Geometry check sheet. Reference: the model listing, model coordinates, mm. A direction names the side the tool comes from. Give positions to 0.01 mm unless a question says otherwise; leave off trailing zeros. Loops run counter-clockwise (first coordinate to the right, second up) from the corner with the lowest first, then second, coordinate; pieces in that order, holes last. Notation, with made-up numbers: (33.5, 61.25) - (80.5, 61.25) arc R25 cw to (80.5, 74.25) - close; hole circle Ø8 at (-25, 49). An arc over 180 degrees is marked (long way). Use a Markdown table: item, result. Add a question column.
1. Cross-section at D-D on y = 9.25. Enter the section's corners in (x, z), and give its area (3 significant figures).
2. Draft check along Z on faces 1 (the flat face through (4, 0, 9)), 2 (the flat face through (2, 10, 2.964)), 3 (the flat face through (4, 10, 27.464)). Enter one of: pulls with the +Z half, pulls with the -Z half, needs draft (parallel to the pull), parting line crosses it, or undercut.
3. Cross-section at B-B on y = 15. Enter the section's corners in (x, z), and give its area (3 significant figures).
4. Cross-section at C-C on z = 16.5. Enter the section's corners in (x, y).
5. Material ranges on L1, parallel to Z at x = 1.75, y = 18.5; L2, parallel to Z at x = 1.75, y = 8.25; L3, parallel to Y at x = 2.5, z = -8, recorded low to high.
6. Cross-section at A-A on x = 3.5. Enter the section's corners in (y, z).
7. Set-up check for faces 4 (the flat face through (0.5, 12, 15)), 5 (the flat face through (2, 10, -5.036)), 6 (the cylindrical face through (3.704, 7.782, 18.618)): record each of +Z, -Z, +X, -X, +Y, -Y from which the full face is reachable in a straight line by a thin tool's end or side.
8. Depth check by flat-ended pin: P1, Ø12, axis at y = 10.5, z = 23, coming from the -X side; P2, Ø2.5, axis at y = 7, z = 0, coming from the -X side; P3, Ø1.5, axis at y = 10, z = 16.5, coming from the +X side. Enter the tip coordinate at first touch or a pass-through.
from build123d import *

# Parameters (mm, degrees)
BOSS_EXTRUDE1_DEPTH = 20
CUT_EXTRUDE1_REACH  = 25.446
SKETCH2_R           = 1.3
SKETCH4_W           = 6.5
SKETCH4_H           = 21.5
BOSS_EXTRUDE2_DEPTH = 20
CUT_EXTRUDE2_REACH  = 36.591
SKETCH6_R           = 1.3
CUT_EXTRUDE3_REACH  = 36.591
SKETCH7_R           = 2.5


with BuildPart() as part:
    # Sketch1 → Boss-Extrude1 (new body)
    with BuildSketch(Plane(origin=(0, 0, 0), x_dir=(-1, 0, 0), z_dir=(0, 1, 0))):
        Polygon((0, -5.035714286), (0, -10.035714286), (-7, -10.035714286), (-7, 5.964285714), (-0.5, 5.964285714), (-0.5, 2.964285714), (-4, 2.964285714), (-4, -5.035714286), align=None)
    extrude(amount=BOSS_EXTRUDE1_DEPTH)

    # Sketch2 → Cut-Extrude1 (cut, up to next)
    with BuildSketch(Plane(origin=(0, 0, 0), x_dir=(0, -1, 0), z_dir=(-1, 0, 0)), mode=Mode.PRIVATE) as cut_extrude1_sk1:
        with Locations(Location((-15, -7.535714286, 0), (0, 0, 90))):
            Circle(SKETCH2_R)
    cut_extrude1_tool1 = extrude(cut_extrude1_sk1.sketch, amount=-CUT_EXTRUDE1_REACH, mode=Mode.PRIVATE) & part.part
    # Sketch2 → Cut-Extrude1 (cut, up to next)
    with BuildSketch(Plane(origin=(0, 0, 0), x_dir=(0, -1, 0), z_dir=(-1, 0, 0)), mode=Mode.PRIVATE) as cut_extrude1_sk2:
        with Locations(Location((-5, -7.535714286, 0), (0, 0, 90))):
            Circle(SKETCH2_R)
    cut_extrude1_tool2 = extrude(cut_extrude1_sk2.sketch, amount=-CUT_EXTRUDE1_REACH, mode=Mode.PRIVATE) & part.part
    add(cut_extrude1_tool1.solids().sort_by_distance((0, 15, -7.535714))[0], mode=Mode.SUBTRACT)
    add(cut_extrude1_tool2.solids().sort_by_distance((0, 5, -7.535714))[0], mode=Mode.SUBTRACT)

    # Sketch4 → Boss-Extrude2 (add)
    with BuildSketch(Plane(origin=(0, 20, 0), x_dir=(-1, 0, 0), z_dir=(0, 1, 0))):
        with Locations((-3.75, 16.714285714)):
            Rectangle(SKETCH4_W, SKETCH4_H)
    extrude(amount=-BOSS_EXTRUDE2_DEPTH)

    # Sketch6 → Cut-Extrude2 (cut, up to next)
    with BuildSketch(Plane(origin=(0.5, 0, 0), x_dir=(0, -1, 0), z_dir=(-1, 0, 0)), mode=Mode.PRIVATE) as cut_extrude2_sk1:
        with Locations(Location((-15, 5.464285714, 0), (0, 0, 90))):
            Circle(SKETCH6_R)
    cut_extrude2_tool1 = extrude(cut_extrude2_sk1.sketch, amount=-CUT_EXTRUDE2_REACH, mode=Mode.PRIVATE) & part.part
    # Sketch6 → Cut-Extrude2 (cut, up to next)
    with BuildSketch(Plane(origin=(0.5, 0, 0), x_dir=(0, -1, 0), z_dir=(-1, 0, 0)), mode=Mode.PRIVATE) as cut_extrude2_sk2:
        with Locations(Location((-5, 5.464285714, 0), (0, 0, 90))):
            Circle(SKETCH6_R)
    cut_extrude2_tool2 = extrude(cut_extrude2_sk2.sketch, amount=-CUT_EXTRUDE2_REACH, mode=Mode.PRIVATE) & part.part
    add(cut_extrude2_tool1.solids().sort_by_distance((0.5, 15, 5.464286))[0], mode=Mode.SUBTRACT)
    add(cut_extrude2_tool2.solids().sort_by_distance((0.5, 5, 5.464286))[0], mode=Mode.SUBTRACT)

    # Sketch7 → Cut-Extrude3 (cut, up to next)
    with BuildSketch(Plane(origin=(0.5, 0, 0), x_dir=(0, -1, 0), z_dir=(-1, 0, 0)), mode=Mode.PRIVATE) as cut_extrude3_sk1:
        with Locations(Location((-10, 17.464285714, 0), (0, 0, 90))):
            Circle(SKETCH7_R)
    cut_extrude3_tool1 = extrude(cut_extrude3_sk1.sketch, amount=-CUT_EXTRUDE3_REACH, mode=Mode.PRIVATE) & part.part
    add(cut_extrude3_tool1.solids().sort_by_distance((0.5, 10, 17.464286))[0], mode=Mode.SUBTRACT)


solid = part.part
Values found:
| question | item | result |
|---|---|---|
| 1 | outline | (0, -10.04) - (7, -10.04) - (7, 15.08) - (0.5, 15.08) - (0.5, 2.96) - (4, 2.96) - (4, -5.04) - (0, -5.04) - close; (0.5, 19.85) - (7, 19.85) - (7, 27.46) - (0.5, 27.46) - close |
| 1 | area | 187 mm2 |
| 2 | face 1 | needs draft |
| 2 | face 2 | undercut |
| 2 | face 3 | pulls with the +Z half |
| 3 | outline | (0, -10.04) - (7, -10.04) - (7, -8.84) - (0, -8.84) - close; (0, -6.24) - (7, -6.24) - (7, 4.16) - (0.5, 4.16) - (0.5, 2.96) - (4, 2.96) - (4, -5.04) - (0, -5.04) - close; (0.5, 6.76) - (7, 6.76) - (7, 27.46) - (0.5, 27.46) - close |
| 3 | area | 183 mm2 |
| 4 | outline | (0.5, 0) - (7, 0) - (7, 7.69) - (0.5, 7.69) - close; (0.5, 12.31) - (7, 12.31) - (7, 20) - (0.5, 20) - close |
| 5 | L1 | z = -10.04 to -5.04, 2.96 to 27.46 |
| 5 | L2 | z = -10.04 to -5.04, 2.96 to 15.68, 19.25 to 27.46 |
| 5 | L3 | y = 0 to 3.79, 6.21 to 13.79, 16.21 to 20 |
| 6 | outline | (0, -10.04) - (20, -10.04) - (20, -5.04) - (0, -5.04) - close; (0, 2.96) - (20, 2.96) - (20, 27.46) - (0, 27.46) - close; hole circle Ø2.6 at (5, -7.54); hole circle Ø2.6 at (5, 5.46); hole circle Ø5 at (10, 17.46); hole circle Ø2.6 at (15, -7.54); hole circle Ø2.6 at (15, 5.46) |
| 7 | face 4 | +Z, -X, +Y, -Y |
| 7 | face 5 | -X, +Y, -Y |
| 7 | face 6 | +X, -X |
| 8 | P1 | stops at x = 0.5 |
| 8 | P2 | stops at x = 4 |
| 8 | P3 | passes through |
